from build123d import *

# Parameters (mm, degrees)
F0_R     = 72
F1_DEPTH = 3
F2_R     = 25.5
F3_DEPTH = 3
F4_R     = 3
F5_DEPTH = 25.4
F6_R     = 3
F7_DEPTH = 25.4


with BuildPart() as f1:
    # F0 (on Top) → F1 (new body)
    with BuildSketch(Plane.XY):
        Circle(F0_R)
    extrude(amount=F1_DEPTH)

    # F2 (on face) → F3 (cut)
    with BuildSketch(Plane.XY.offset(3)):
        with Locations((-40.5, 0)):
            Circle(F2_R)
        with Locations((40.5, 0)):
            Circle(F2_R)
    extrude(amount=-F3_DEPTH, mode=Mode.SUBTRACT)

    # F4 (on face) → F5 (cut)
    with BuildSketch(Plane.XY.offset(3)):
        with Locations((0, 61.5)):
            Circle(F4_R)
        Circle(F4_R)
        with Locations((0, -61.5)):
            Circle(F4_R)
    extrude(amount=-F5_DEPTH, mode=Mode.SUBTRACT)

    # F6 (on face) → F7 (cut)
    with BuildSketch(Plane.XY.offset(3)):
        with Locations((-53.260562, -30.75)):
            Circle(F6_R)
        with Locations((53.260562, -30.75)):
            Circle(F6_R)
    extrude(amount=-F7_DEPTH, mode=Mode.SUBTRACT)


solid = f1.part
Verification items for the finished model (mm, model axes). Coordinates: 2 decimals unless noted, no trailing zeros. Write each loop counter-clockwise with the first axis right and the second up, starting at its lowest first coordinate (ties: lowest second). Pieces come first, ordered by that corner, then holes. Notation, with made-up numbers: (47.5, -4.75) -> (106.5, -4.75) arc R17 cw to (106.5, 11.25) -> close; hole circle Ø3 at (54, -39). An arc over 180 degrees is marked (long way). One line per item, written item: value. Start each with the question number.
Q1. Mould release check, pull along X, two halves, no side actions. Record for faces 1 (the flat face through (-1, -15, 0)), 2 (the cylindrical face through (-9.373, 71.387, 1.479)), 3 (the cylindrical face through (-56.258, -30.618, 1.521)), 4 (the cylindrical face through (-0.391, -58.526, 1.521)): pulls with the +X half, pulls with the -X half, needs draft (parallel to the pull), parting line crosses it, or undercut.
Q2. Thickness scan on L1, parallel to Y at x = 2.5, z = 1.1; L2, parallel to Y at x = 54, z = 1.9; L3, parallel to Y at x = -55.5, z = 2.5. Record the ranges inside material, lowest first. Write a range as from..to.
Q3. Cross-section at C-C on z = 1.85. Enter the section's corners in (x, y), and give its area (3 significant figures).
Q4. Cross-section at D-D on x = 40.5. Enter the section's corners in (y, z).
Q5. Cross-section at B-B on y = 0. Enter the section's corners in (x, z).
Q6. Go/stop test with flat-tipped pins: P1, Ø1.5, axis at y = -19, z = 2, coming from the +X side; P2, Ø5, axis at x = 55.5, y = -52, coming from the -Z side (3 decimals). Record where each tip stops, or that it passes through.
Q7. Cross-section at A-A on x = 0. Enter the section's corners in (y, z).
Checked values:
1. face 1: needs draft
1. face 2: parting line crosses it
1. face 3: undercut
1. face 4: undercut
2. L1: y = -71.96..-63.16, -59.84..-1.66, 1.66..59.84, 63.16..71.96
2. L2: y = -47.62..-33.66, -27.84..-21.63, 21.63..47.62
2. L3: y = -45.87..-32.75, -28.75..-20.62, 20.62..45.87
3. outline: circle Ø144 at (0, 0); hole circle Ø51 at (-40.5, 0); hole circle Ø6 at (-53.26, -30.75); hole circle Ø6 at (0, -61.5); hole circle Ø6 at (0, 0); hole circle Ø6 at (0, 61.5); hole circle Ø51 at (40.5, 0); hole circle Ø6 at (53.26, -30.75)
3. area: 12,100 mm²
4. outline: (-59.53, 0) -> (-25.5, 0) -> (-25.5, 3) -> (-59.53, 3) -> close; (25.5, 0) -> (59.53, 0) -> (59.53, 3) -> (25.5, 3) -> close
5. outline: (-72, 0) -> (-66, 0) -> (-66, 3) -> (-72, 3) -> close; (-15, 0) -> (-3, 0) -> (-3, 3) -> (-15, 3) -> close; (3, 0) -> (15, 0) -> (15, 3) -> (3, 3) -> close; (66, 0) -> (72, 0) -> (72, 3) -> (66, 3) -> close
6. P1: stops at x = 69.65
6. P2: passes through
7. outline: (-72, 0) -> (-64.5, 0) -> (-64.5, 3) -> (-72, 3) -> close; (-58.5, 0) -> (-3, 0) -> (-3, 3) -> (-58.5, 3) -> close; (3, 0) -> (58.5, 0) -> (58.5, 3) -> (3, 3) -> close; (64.5, 0) -> (72, 0) -> (72, 3) -> (64.5, 3) -> close
